Model file for the job. Use its own axes, mm. A direction names the side the tool comes from. Coordinates: 2 decimals unless noted, no trailing zeros. Write each loop counter-clockwise with the first axis right and the second up, starting at its lowest first coordinate (ties: lowest second). Pieces come first, ordered by that corner, then holes. Notation, with made-up numbers: (72, 81.5) - (89, 81.5) arc R29 ccw to (89, 116.5) - close; hole circle Ø11 at (1, 3). An arc over 180 degrees is marked (long way). Put each result on its own line as item: value. Start each with the question number.
1. Saw through at A-A, the plane x = 7.75. Write the cut outline in (y, z), plus the area to 3 significant figures.
2. Drop flat-ended pins along their axis: P1, Ø1.1, axis at y = 18.5, z = 3.5, coming from the +X side; P2, Ø3, axis at y = 10, z = 4.5, coming from the +X side; P3, Ø4, axis at y = 29.5, z = 3, coming from the +X side. Give the stop position or say it passes through.
3. Saw through at B-B, the plane z = 2.5. Write the cut outline in (x, y), plus the area to 3 significant figures.
4. Saw through at C-C, the plane y = 26. Write the cut outline in (x, z), plus the area to 3 significant figures.
5. Drill centre lines: L1, parallel to Y at x = 20.25, z = 1; L2, parallel to X at y = 3, z = 1.75; L3, parallel to X at y = 34, z = 0.5. Where is each one in solid material? Low to high. Write a range as from..to.
6. Which spindle directions (+Z, -Z, +X, -X, +Y, -Y) get a long thin tool onto all of the face, cutting with end or side? Do faces 1 (the face through (5, 18, 4)), 2 (the face through (25, 1, 4)). Say none if no direction does.
7. Saw through at D-D, the plane y = 6.9. Write the cut outline in (x, z).
```python
from build123d import *

# Parameters (mm, degrees)
BOSS_EXTRUDE1_DEPTH = 8
SKETCH1_3_R         = 1.9
BOSS_EXTRUDE2_DEPTH = 8
LPATTERN1_COUNT     = 5
LPATTERN1_PITCH     = 7.6
CHAMFER1_SIZE       = 3


with BuildPart() as part:
    # Sketch1 → Boss-Extrude1 (new body)
    with BuildSketch(Plane.XY):
        Polygon((0, 0), (0, 48), (25, 48), (25, 43), (5, 43), (5, 5), (25, 5), (25, 0), align=None)
    extrude(amount=BOSS_EXTRUDE1_DEPTH)

    # Sketch1<3> → Boss-Extrude2 (add)
    with BuildSketch(Plane.XY):
        with Locations((5, 6.9)):
            Circle(SKETCH1_3_R)
    boss_extrude2 = extrude(amount=BOSS_EXTRUDE2_DEPTH)

    # LPattern1: Boss-Extrude2 ×5
    with Locations(*[(0, i * LPATTERN1_PITCH, 0) for i in range(1, LPATTERN1_COUNT)]):
        add(boss_extrude2)

    # Chamfer1
    chamfer1_edges = [part.edges().sort_by_distance(p)[0] for p in [
        (25, 43, 4),
        (25, 5, 4),
    ]]
    chamfer(chamfer1_edges, length=CHAMFER1_SIZE)


solid = part.part
```
Final values:
1. outline: (0, 0) - (5, 0) - (5, 8) - (0, 8) - close; (43, 0) - (48, 0) - (48, 8) - (43, 8) - close
1. area: 80.0 mm²
2. P1: stops at x = 5
2. P2: stops at x = 6.02
2. P3: stops at x = 6.9
3. outline: (0, 0) - (25, 0) - (25, 2) - (22, 5) - (5, 5) arc R1.9 ccw to (5, 8.8) - (5, 12.6) arc R1.9 ccw to (5, 16.4) - (5, 20.2) arc R1.9 ccw to (5, 24) - (5, 27.8) arc R1.9 ccw to (5, 31.6) - (5, 35.4) arc R1.9 ccw to (5, 39.2) - (5, 43) - (22, 43) - (25, 46) - (25, 48) - (0, 48) - close
3. area: 459 mm²
4. outline: (0, 0) - (5, 0) - (5, 8) - (0, 8) - close
4. area: 40.0 mm²
5. L1: y = 0..5, 43..48
5. L2: x = 0..24
5. L3: x = 0..5
6. face 1: +Z, -Z, +X
6. face 2: +Z, -Z, +X, +Y, -Y
7. outline: (0, 0) - (6.9, 0) - (6.9, 8) - (0, 8) - close
